```python
from build123d import *

# Parameters (mm, degrees)
SKETCH2_R           = 5.7
CUT_EXTRUDE1_DEPTH  = 52.923019943
BOSS_EXTRUDE1_START = 2
SKETCH3_R           = 8
SKETCH3_R_2         = 5.7
BOSS_EXTRUDE1_DEPTH = 2
SKETCH4_R           = 8
SKETCH4_R_2         = 5.7
BOSS_EXTRUDE2_DEPTH = 2


with BuildPart() as part:
    # Sketch1 → Revolve1 (revolve)
    with BuildSketch(Plane.XY, mode=Mode.PRIVATE) as revolve1_sk:
        Polygon((-24, 0), (24, 0), (24, 14), (22, 14), (22, 6.7), (-22, 6.7), (-22, 14), (-24, 14), align=None)
    revolve(revolve1_sk.sketch.rotate(Axis((-24, 0, 0), (1, 0, 0)), 180), axis=Axis((-24, 0, 0), (1, 0, 0)))

    # Sketch2 → Cut-Extrude1 (cut, through all)
    with BuildSketch(Plane(origin=(24, 0, 0), x_dir=(0, 0, -1), z_dir=(1, 0, 0))):
        Circle(SKETCH2_R)
    extrude(amount=-CUT_EXTRUDE1_DEPTH, mode=Mode.SUBTRACT)

    # Sketch3 → Boss-Extrude1 (add)
    with BuildSketch(Plane(origin=(24, 0, 0), x_dir=(0, 0, -1), z_dir=(1, 0, 0)).offset(BOSS_EXTRUDE1_START)):
        with Locations(Location((0, 0, 0), (0, 0, 270))):
            Circle(SKETCH3_R)
        Circle(SKETCH3_R_2, mode=Mode.SUBTRACT)
    extrude(amount=-BOSS_EXTRUDE1_DEPTH)

    # Sketch4 → Boss-Extrude2 (add)
    with BuildSketch(Plane.ZY.offset(24)):
        with Locations(Location((0, 0, 0), (0, 0, 270))):
            Circle(SKETCH4_R)
        with Locations(Location((0, 0, 0), (0, 0, 180))):
            Circle(SKETCH4_R_2, mode=Mode.SUBTRACT)
    extrude(amount=BOSS_EXTRUDE2_DEPTH)


solid = part.part
```
Geometry check sheet. Reference: the model listing, model coordinates, mm. A direction names the side the tool comes from. Round coordinates to 2 decimals unless told otherwise and drop trailing zeros. Loops run counter-clockwise (first coordinate to the right, second up) from the corner with the lowest first, then second, coordinate; pieces in that order, holes last. Notation, with made-up numbers: M 64,49 L 118,49 A22 cw 118,64 Z; hole C 32,-27.75 d4. An arc over 180 degrees is marked long. Return JSON: item names as keys, results as strings. Group by question number.
(1) Go/stop test with flat-tipped pins: pin 1 (10 mm diameter, centred on x = 3, z = 2.5, fed in from -Y); pin 2 (3 mm diameter, centred on x = -5.5, y = -1.5, fed in from +Z); pin 3 (4 mm diameter, centred on x = 0.5, y = -6, fed in from +Z). Record where each tip stops, or that it passes through.
(2) Set-up check for faces 1 (the face through (-24.99, 1.73, -7.81)), 2 (the face through (24, 6, 6)), 3 (the face through (-0.31, 1.45, 6.54)): record each of +Z, -Z, +X, -X, +Y, -Y from which the full face is reachable in a straight line by a thin tool's end or side.
(3) Section check A-A, the plane y = 0. Enter the section's corners in (x, z).
(4) Section check D-D, the plane y = -10.5. Enter the section's corners in (x, z), and give its area (3 significant figures).
(5) Section check C-C, the plane x = 6. Enter the section's corners in (y, z).
(6) Section check B-B, the plane z = -3. Enter the section's corners in (x, y), and give its area (3 significant figures).
(7) Scan lines: line 1 along X through (y, z) = (5.75, 8.25); line 2 along Z through (x, y) = (0, 0); line 3 along Y through (x, z) = (14, 3.75). Record each from-to range of solid material in increasing order. Write a range as [from, to].
(8) Mould release check, pull along Z, two halves, no side actions. Record for faces 4 (the face through (22.986, -12.932, 5.362)), 5 (the face through (0.364, 5.564, 1.236)), 6 (the face through (-24, -6, 6)): pulls with the +Z half, pulls with the -Z half, needs draft (parallel to the pull), parting line crosses it, or undercut.
Data:
{
 "1": {"pin 1": "y = -6.7", "pin 2": "z = 6.7", "pin 3": "z = 5.37"},
 "2": {"face 1": "-X", "face 2": "+X", "face 3": "none"},
 "3": {"outline": "M -26,-8 L -24,-8 L -24,-14 L -22,-14 L -22,-6.7 L 22,-6.7 L 22,-14 L 24,-14 L 24,-8 L 26,-8 L 26,-5.7 L -26,-5.7 Z; M -26,5.7 L 26,5.7 L 26,8 L 24,8 L 24,14 L 22,14 L 22,6.7 L -22,6.7 L -22,14 L -24,14 L -24,8 L -26,8 Z"},
 "4": {"outline": "M -24,-9.26 L -22,-9.26 L -22,9.26 L -24,9.26 Z; M 22,-9.26 L 24,-9.26 L 24,9.26 L 22,9.26 Z", "area": "74.1 mm²"},
 "5": {"outline": "C 0,0 d13.4; hole C 0,0 d11.4"},
 "6": {"outline": "M -26,-7.42 L -24,-7.42 L -24,-13.67 L -22,-13.67 L -22,-5.99 L 22,-5.99 L 22,-13.67 L 24,-13.67 L 24,-7.42 L 26,-7.42 L 26,-4.85 L -26,-4.85 Z; M -26,4.85 L 26,4.85 L 26,7.42 L 24,7.42 L 24,13.67 L 22,13.67 L 22,5.99 L -22,5.99 L -22,13.67 L -24,13.67 L -24,7.42 L -26,7.42 Z", "area": "192 mm²"},
 "7": {"line 1": "[-24, -22], [22, 24]", "line 2": "[-6.7, -5.7], [5.7, 6.7]", "line 3": "[-5.55, -4.29], [4.29, 5.55]"},
 "8": {"face 4": "parting line crosses it", "face 5": "undercut", "face 6": "needs draft"}
}
